```python
from build123d import *

# Parameters (mm, degrees)
BOSS_EXTRUDE1_DEPTH = 15
CUT_EXTRUDE1_START  = -1.6
CUT_EXTRUDE1_DEPTH  = 11.8
SKETCH3_R           = 1.9
CUT_EXTRUDE2_DEPTH  = 31.805843601
SKETCH4_R           = 1.9
CUT_EXTRUDE3_DEPTH  = 31.805843601


with BuildPart() as part:
    # Sketch1 → Boss-Extrude1 (new body)
    with BuildSketch(Plane.XY):
        Polygon((0, 0), (-20, 0), (0, 20), align=None)
    extrude(amount=BOSS_EXTRUDE1_DEPTH)

    # Sketch2 → Cut-Extrude1 (cut)
    with BuildSketch(Plane.XY.offset(15).offset(CUT_EXTRUDE1_START)):
        Polygon((-18, 2), (-2, 18), (-2, 2), align=None)
    extrude(amount=-CUT_EXTRUDE1_DEPTH, mode=Mode.SUBTRACT)

    # Sketch3 → Cut-Extrude2 (cut, through all)
    with BuildSketch(Plane.ZY.offset(2)):
        with Locations(Location((7.5, 9.6, 0), (0, 0, 270))):
            Circle(SKETCH3_R)
    extrude(amount=-CUT_EXTRUDE2_DEPTH, mode=Mode.SUBTRACT)

    # Sketch4 → Cut-Extrude3 (cut, through all)
    with BuildSketch(Plane(origin=(0, 2, 0), x_dir=(1, 0, 0), z_dir=(0, 1, 0))):
        with Locations(Location((-9.6, -7.5, 0), (0, 0, 180))):
            Circle(SKETCH4_R)
    extrude(amount=-CUT_EXTRUDE3_DEPTH, mode=Mode.SUBTRACT)


solid = part.part
```
Verification items for the finished model (mm, model axes). A direction names the side the tool comes from. Give positions to 0.01 mm unless a question says otherwise; leave off trailing zeros. Order: outer loops, then holes, each group sorted by start corner. A loop starts at its lowest first (then second) coordinate and runs counter-clockwise, first axis right, second up. Notation, with made-up numbers: M 30,-26.75 L 78,-26.75 A8 ccw 78,-11.75 Z; hole C 46.25,-27 d7. An arc over 180 degrees is marked long. Return JSON: item names as keys, results as strings. Group by question number.
1) Go/stop test with a flat-tipped pin: pin 1 Ø5 at (y, z) = (9.6, 7.5) entering from -X. Record where the tip stops, or that it passes through.
2) Scan lines: line 1 (Z direction, x = -4, y = 15.75); line 2 (Z direction, x = -0.65, y = 9.6); line 3 (X direction, y = 17.25, z = 5.5). Record each from-to range of solid material in increasing order.
3) Section check C-C on y = 11. Record the cut outline in (x, z).
4) Section check B-B on x = -9.6. Record the cut outline in (y, z).
5) Mould release check, pull along Z, two halves, no side actions. Record for faces 3 (the face through (-5, 6, 0)), 4 (the face through (-2, 12, 8)), 5 (the face through (0, 12, 7)): pulls with the +Z half, pulls with the -Z half, needs draft (parallel to the pull), parting line crosses it, or undercut.
6) Access from +Z, -Z, +X, -X, +Y, -Y to the whole of each face (thin tool, end or side, straight path). Record for faces 1 (the face through (-5, 6, 15)), 2 (the face through (-12, 2, 8)).
7) Section check D-D on y = 6.75. Record the cut outline in (x, z).
8) Section check A-A on z = 7.5. Record the cut outline in (x, y).
Answer block:
{
 "1": {"pin 1": "stops at x = -2"},
 "2": {"line 1": "z = 0 to 1.6, 13.4 to 15", "line 2": "z = 0 to 5.6, 9.4 to 15", "line 3": "x = -2 to 0"},
 "3": {"outline": "M -9,0 L 0,0 L 0,6.22 L -2,6.22 L -2,1.6 L -9,1.6 Z; M -9,13.4 L -2,13.4 L -2,8.78 L 0,8.78 L 0,15 L -9,15 Z"},
 "4": {"outline": "M 0,0 L 10.4,0 L 10.4,1.6 L 2,1.6 L 2,5.6 L 0,5.6 Z; M 0,9.4 L 2,9.4 L 2,13.4 L 10.4,13.4 L 10.4,15 L 0,15 Z"},
 "5": {"face 3": "pulls with the -Z half", "face 4": "undercut", "face 5": "needs draft"},
 "6": {"face 1": "+Z, +X, -X, +Y, -Y", "face 2": "-X, +Y"},
 "7": {"outline": "M -13.25,0 L 0,0 L 0,15 L -13.25,15 L -13.25,13.4 L -2,13.4 L -2,1.6 L -13.25,1.6 Z"},
 "8": {"outline": "M -20,0 L -11.5,0 L -11.5,2 L -18,2 Z; M -7.7,0 L 0,0 L 0,7.7 L -2,7.7 L -2,2 L -7.7,2 Z; M -2,11.5 L 0,11.5 L 0,20 L -2,18 Z"}
}
